Can you work these out from the drawing? Everything is in mm from the part's minimum corner. A direction names the side the tool comes from. Coordinates: 2 decimals unless noted, no trailing zeros. Order: outer loops, then holes, each group sorted by start corner. A loop starts at its lowest first (then second) coordinate and runs counter-clockwise, first axis right, second up. Notation, with made-up numbers: (-32.75, -39) -> (12.25, -39) arc R14 cw to (12.25, -28) -> close; hole circle Ø5 at (87.5, 69). An arc over 180 degrees is marked (long way). Return JSON: item names as keys, results as strings. Group by question number.
1) If we section it at C-C, the plane y = 3: Please give me the cut outline in (x, z).
2) If we section it at B-B, the plane x = 24: Please give me the cut outline in (y, z).
3) For pin 1 (1.5 mm diameter, centred on y = 4.5, z = 1.5, fed in from +X), with a flat end and sliding along its axis, tell me the tip position at first contact or that it passes through.
4) If I drill on probe 1 along Y at (x, z) = (24, 5.6); probe 2 along X at (y, z) = (4.75, 4); probe 3 along Z at (x, y) = (3.75, 3.5), over which ranges is the centre line in solid material (lowest first)? Write a range as from..to.
5) Thinking about a two-plate mould opening in Y: for the marked faces 1, 2 and 3, which applies, +Y half, -Y half, draft (parallel to the pull), parting line (faces both ways), or undercut?
6) If we section it at D-D, the plane x = 6.75: Please give me the cut outline in (y, z), then the cut area to 3 significant figures.
7) If we section it at A-A, the plane z = 6.25: Please give me the cut outline in (x, y).
8) For the marked faces 4, 5 and 6, which set-ups out of +Z, -Z, +X, -X, +Y, -Y let a thin tool reach every point of the face, with its end or its side?
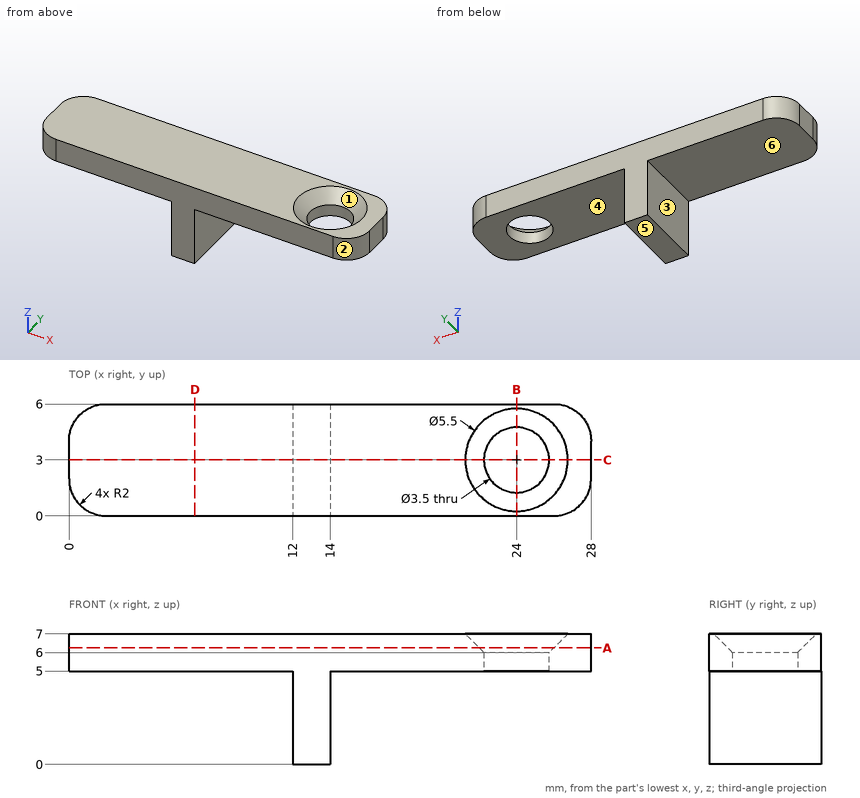
Result sheet:
{
 "1": {"outline": "(0, 5) -> (12, 5) -> (12, 0) -> (14, 0) -> (14, 5) -> (22.25, 5) -> (22.25, 6) -> (21.25, 7) -> (0, 7) -> close; (25.75, 5) -> (28, 5) -> (28, 7) -> (26.75, 7) -> (25.75, 6) -> close"},
 "2": {"outline": "(0, 5) -> (1.25, 5) -> (1.25, 6) -> (0.25, 7) -> (0, 7) -> close; (4.75, 5) -> (6, 5) -> (6, 7) -> (5.75, 7) -> (4.75, 6) -> close"},
 "3": {"pin 1": "stops at x = 14"},
 "4": {"probe 1": "y = 0..1.25, 4.75..6", "probe 2": "x = 12..14", "probe 3": "z = 5..7"},
 "5": {"face 1": "undercut", "face 2": "-Y half", "face 3": "draft"},
 "6": {"outline": "(0, 5) -> (6, 5) -> (6, 7) -> (0, 7) -> close", "area": "12.0 mm2"},
 "7": {"outline": "(0, 2) arc R2 ccw to (2, 0) -> (26, 0) arc R2 ccw to (28, 2) -> (28, 4) arc R2 ccw to (26, 6) -> (2, 6) arc R2 ccw to (0, 4) -> close; hole circle Ø4 at (24, 3)"},
 "8": {"face 4": "-Z, +X, +Y, -Y", "face 5": "-Z, +X, -X, +Y, -Y", "face 6": "-Z, -X, +Y, -Y"}
}
